Design review of the part built by this model. Coordinates are the model's own, in mm. Give positions to 0.01 mm unless a question says otherwise; leave off trailing zeros. Loops run counter-clockwise (first coordinate to the right, second up) from the corner with the lowest first, then second, coordinate; pieces in that order, holes last. Notation, with made-up numbers: (-26.5, 29) -> (-9.5, 29) arc R18 cw to (-9.5, 34) -> close; hole circle Ø3 at (-20.5, 43). An arc over 180 degrees is marked (long way). Use CSV: the item, a comma, the result in double quotes. Start each with the question number.
Item 1: Wall thickness on line 1 along Y through (x, z) = (-23, 1.65); line 2 along X through (y, z) = (9.5, 0.9); line 3 along X through (y, z) = (18, 1.75): over which ranges is each line inside the solid? List them lowest first. Write a range as from..to.
Item 2: Clearance check with flat-ended pins moving along their axes: pin 1 (1.2 mm diameter, centred on x = 24, z = 1.5, fed in from -Y); pin 2 (1.5 mm diameter, centred on x = 16.5, z = 3, fed in from +Y); pin 3 (2 mm diameter, centred on x = 22.5, z = 3.5, fed in from +Y). State where each tip first meets the part, or that it passes through.
Item 3: We need section A-A (y = -1). State the section outline as (x, z) points.
Item 4: We need section C-C (z = 2.05). Count the separate pieces of the cut face and the enclosed holes in it, plus the area to 3 significant figures.
Item 5: We need section D-D (y = -50). State the section outline as (x, z) points.
Item 6: We need section B-B (y = 15). State the section outline as (x, z) points.
from build123d import *

# Parameters (mm, degrees)
F1_DEPTH = 4


with BuildPart() as f1:
    # F0 (on Top) → F1 (new body)
    with BuildSketch(Plane.XY):
        with BuildLine():
            Line((-9.863807, -65.836951), (-28.221913, -70.849411))
            Line((-28.221913, -70.849411), (-5.88068, -70.849411))
            Line((-5.88068, -70.849411), (5.52761, -51.597916))
            Line((5.52761, -51.597916), (22.877717, -56.113698))
            Line((22.877717, -56.113698), (16.460553, -71.562424))
            Line((16.460553, -71.562424), (30.720916, -54.44999))
            Line((30.720916, -54.44999), (11.707101, -47.319807))
            Line((11.707101, -47.319807), (18.559989, -19.489294))
            Line((18.559989, -19.489294), (27.928099, -17.142748))
            Line((27.928099, -17.142748), (31.150259, -20.496517))
            Line((31.150259, -20.496517), (29.922873, -16.418136))
            Line((29.922873, -16.418136), (40.215254, 6.320762))
            ThreePointArc((40.215254, 6.320762), (39.07685, 4.638557), (37.845484, 3.023156))
            Line((37.845484, 3.023156), (30.833699, 10.89257))
            Line((30.833699, 10.89257), (37.233405, 13.086755))
            Line((37.233405, 13.086755), (41.796244, 9.064083))
            ThreePointArc((41.796244, 9.064083), (45.083627, 18.276724), (45.772686, 28.03402))
            Line((45.772686, 28.03402), (41.621767, 22.594886))
            Line((41.621767, 22.594886), (38.548019, 28.587904))
            Line((38.548019, 28.587904), (32.479335, 31.188771))
            Line((32.479335, 31.188771), (27.359569, 28.628892))
            Line((27.359569, 28.628892), (20.41132, 33.931505))
            Line((20.41132, 33.931505), (7.97761, 29.908832))
            Line((7.97761, 29.908832), (20.41132, 39.051265))
            Line((20.41132, 39.051265), (25.165388, 39.051265))
            Line((25.165388, 39.051265), (26.628176, 43.622486))
            Line((26.628176, 43.622486), (22.788357, 41.336875))
            Line((22.788357, 41.336875), (20.41132, 45.33029))
            Line((20.41132, 45.33029), (15.657255, 39.051265))
            Line((15.657255, 39.051265), (19.131379, 51.119279))
            Line((19.131379, 51.119279), (28.63951, 45.450971))
            Line((28.63951, 45.450971), (38.112831, 47.983287))
            ThreePointArc((38.112831, 47.983287), (24.277711, 58.679623), (7.036208, 61.604132))
            Line((7.036208, 61.604132), (4.686333, 44.171032))
            Line((4.686333, 44.171032), (-1.90921, 54.959098))
            Line((-1.90921, 54.959098), (-1.90921, 59.75246))
            ThreePointArc((-1.90921, 59.75246), (-10.497436, 55.445101), (-17.642448, 49.021725))
            Line((-17.642448, 49.021725), (-11.221501, 50.387885))
            Line((-11.221501, 50.387885), (-9.393012, 41.793998))
            Line((-9.393012, 41.793998), (-6.284588, 50.570734))
            Line((-6.284588, 50.570734), (1.943606, 46.365213))
            Line((1.943606, 46.365213), (-3.17616, 43.439634))
            Line((-3.17616, 43.439634), (-6.833133, 27.897498))
            Line((-6.833133, 27.897498), (-8.47877, 32.285865))
            Line((-8.47877, 32.285865), (-19.998237, 30.457377))
            Line((-19.998237, 30.457377), (-17.804054, 25.337616))
            Line((-17.804054, 25.337616), (-24.386607, 30.274531))
            Line((-24.386607, 30.274531), (-21.09533, 35.942841))
            Line((-21.09533, 35.942841), (-23.083921, 40.398134))
            ThreePointArc((-23.083921, 40.398134), (-24.639853, 15.082316), (-9.133734, -4.989351))
            Line((-9.133734, -4.989351), (0.724342, -27.495166))
            Line((0.724342, -27.495166), (9.211371, -22.117248))
            Line((9.211371, -22.117248), (1.528105, -46.750505))
            Line((1.528105, -46.750505), (-9.863807, -65.836951))
        make_face()
        with BuildLine():
            ThreePointArc((-7.636228, -5.865513), (7.079238, -10.265979), (22.290661, -8.13956))
            Line((22.290661, -8.13956), (9.517227, -17.271729))
            Line((9.517227, -17.271729), (2.47791, -21.973379))
            Line((2.47791, -21.973379), (-7.636228, -5.865513))
        make_face(mode=Mode.SUBTRACT)
        Polygon((23.370633, -12.399131), (24.836801, -13.925185), (19.892599, -15.154307), align=None, mode=Mode.SUBTRACT)
        Polygon((-16.524114, 17.292272), (-24.752304, 23.874825), (-10.855804, 21.863492), (-15.061324, 1.567287), align=None, mode=Mode.SUBTRACT)
        Polygon((25.768461, 6.672658), (22.971205, 9.064083), (24.597929, 12.859768), align=None, mode=Mode.SUBTRACT)
        Polygon((24.433995, 19.12076), (19.497076, 7.601293), (16.937198, 21.132095), (9.809952, 25.670725), (19.497076, 31.554472), (25.165388, 25.703313), align=None, mode=Mode.SUBTRACT)
        with BuildLine():
            Line((28.05753, -10.219939), (26.818711, -6.103566))
            ThreePointArc((26.818711, -6.103566), (32.490768, -2.337917), (37.353444, 2.427242))
            Line((37.353444, 2.427242), (28.05753, -10.219939))
        make_face(mode=Mode.SUBTRACT)
    extrude(amount=F1_DEPTH)


solid = f1.part
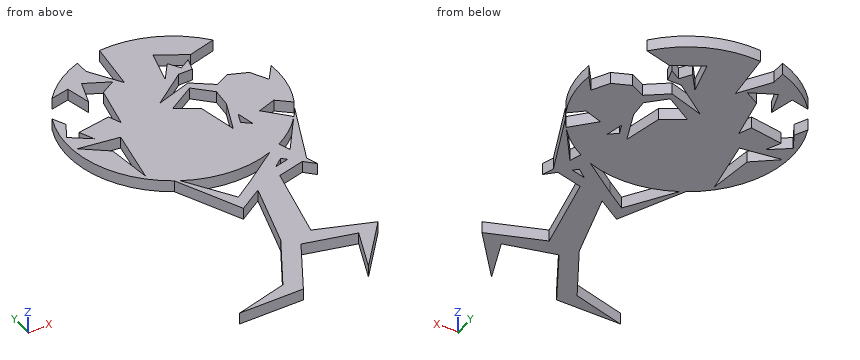
Results found:
1,line 1,"-70.85..-69.42, 10.76..22.47, 23.62..29.23, 32.66..40.21"
1,line 2,"-22.4..-15.8, -13.42..19.14, 20.31..23.16, 25.23..32.07, 41.3..42.02"
1,line 3,"-25.4..-17.41, -11.66..17.53, 23.95..45.02"
2,pin 1,"y = -63.24"
2,pin 2,"y = 61.22"
2,pin 3,"y = 59.76"
3,outline,"(-14.43, 0) -> (34.05, 0) -> (34.05, 4) -> (-14.43, 4) -> close; (34.83, 0) -> (36.9, 0) -> (36.9, 4) -> (34.83, 4) -> close"
4,separate pieces,"1"
4,enclosed holes,"6"
4,area,"3,820 mm²"
5,outline,"(-0.41, 0) -> (18.85, 0) -> (18.85, 4) -> (-0.41, 4) -> close"
6,outline,"(-24.61, 0) -> (-16.31, 0) -> (-16.31, 4) -> (-24.61, 4) -> close; (-12.28, 0) -> (18.1, 0) -> (18.1, 4) -> (-12.28, 4) -> close; (22.67, 0) -> (44.23, 0) -> (44.23, 4) -> (22.67, 4) -> close"
